from build123d import *

# Parameters (mm, degrees)
SKETCH_1_W            = 20
SKETCH_1_H            = 25
EXTRUDE_1_DEPTH       = 2
SKETCH_2_W            = 18.5
SKETCH_2_H            = 6
EXTRUDE_2_DEPTH       = 15
SKETCH_3_W            = 10
SKETCH_3_H            = 12
CUT_EXTRUDE_1_DEPTH   = 30.618406439
HOLE_WIZARD_3_0_3_1_D = 3


with BuildPart() as part:
    # 草圖1 → 填料-伸長1 (new body)
    with BuildSketch(Plane.XZ.offset(2)):
        with Locations((0, 11)):
            Rectangle(SKETCH_1_W, SKETCH_1_H)
    extrude(amount=-EXTRUDE_1_DEPTH)

    # 草圖2 → 填料-伸長2 (add)
    with BuildSketch(Plane(origin=(0, 0, 0), x_dir=(-1, 0, 0), z_dir=(0, 1, 0))):
        with Locations((0, 3)):
            Rectangle(SKETCH_2_W, SKETCH_2_H)
    extrude(amount=EXTRUDE_2_DEPTH)

    # 草圖3 → 除料-伸長1 (cut, through all)
    with BuildSketch(Plane(origin=(0, 0, 0), x_dir=(-1, 0, 0), z_dir=(0, 0, -1))):
        with Locations((0, 9)):
            Rectangle(SKETCH_3_W, SKETCH_3_H)
    extrude(amount=-CUT_EXTRUDE_1_DEPTH, mode=Mode.SUBTRACT)

    # Ø3.0 (3) 直徑孔1 (through all)
    with Locations(Plane(origin=(0, 0, 0), x_dir=(1, 0, 0), z_dir=(0, 1, 0))):
        with Locations((-7.5, -21), (7.5, -21)):
            Hole(HOLE_WIZARD_3_0_3_1_D / 2)


solid = part.part
The model under review builds one solid part; all positions refer to its coordinate system, in mm. A direction names the side the tool comes from. Give positions to 0.01 mm unless a question says otherwise; leave off trailing zeros. Write each loop counter-clockwise with the first axis right and the second up, starting at its lowest first coordinate (ties: lowest second). Pieces come first, ordered by that corner, then holes.
1. Draft analysis for pull direction Z (two halves, no side actions). For faces 1 (the flat face through (0, 0, 14)), 2 (the flat face through (0, 2, 0)), 3 (the cylindrical face through (-6.39, -1.01, 19.99)), state which applies: +Z half, -Z half, draft (parallel to the pull), parting line (faces both ways), or undercut.
2. Add section A-A, the plane x = 7.5. Write out the cut boundary in (y, z).
3. For P1, Ø2, axis at x = -4, y = 2, coming from the -Z side; P2, Ø5, axis at y = 6, z = 2, coming from the +X side; P3, Ø5, axis at y = 6, z = 4, coming from the -X side; P4, Ø6.5, axis at x = -2, z = 4, coming from the +Y side, all flat-tipped, find the tip position at first contact; note any pin that passes through.
4. Add section C-C, the plane y = 13. Write out the cut boundary in (x, z), plus the area to 3 significant figures.
5. Add section D-D, the plane z = 5. Write out the cut boundary in (x, y).
6. Tool access review of faces 4 (the flat face through (9.25, 7, 3)), 5 (the flat face through (-9.25, 7, 3)), 6 (the flat face through (5, 9, 3)), 7 (the flat face through (0, 2, 6)): name each direction out of +Z, -Z, +X, -X, +Y, -Y from which nothing blocks a thin tool from reaching the whole face with its end or side.
7. Wall thickness on L1, parallel to X at y = -1, z = 21; L2, parallel to X at y = 13.25, z = 5.5; L3, parallel to Z at x = 7.5, y = -1.1: over which ranges is each line inside the solid? List them lowest first.
8. Add section B-B, the plane z = 21. Write out the cut boundary in (x, y).
Worked answers:
1. face 1: draft
1. face 2: -Z half
1. face 3: undercut
2. outline: (-2, -1.5) - (0, -1.5) - (0, 0) - (15, 0) - (15, 6) - (0, 6) - (0, 19.5) - (-2, 19.5) - close; (-2, 22.5) - (0, 22.5) - (0, 23.5) - (-2, 23.5) - close
3. P1: stops at z = 0
3. P2: stops at x = 9.25
3. P3: stops at x = -9.25
3. P4: stops at y = 15
4. outline: (-9.25, 0) - (-5, 0) - (-5, 6) - (-9.25, 6) - close; (5, 0) - (9.25, 0) - (9.25, 6) - (5, 6) - close
4. area: 51.0 mm2
5. outline: (-10, -2) - (10, -2) - (10, 0) - (9.25, 0) - (9.25, 15) - (5, 15) - (5, 3) - (-5, 3) - (-5, 15) - (-9.25, 15) - (-9.25, 0) - (-10, 0) - close
6. face 4: +Z, -Z, +X, +Y
6. face 5: +Z, -Z, -X, +Y
6. face 6: +Z, -Z, +Y
6. face 7: +Z, +X, -X, +Y
7. L1: x = -10 to -9, -6 to 6, 9 to 10
7. L2: x = -9.25 to -5, 5 to 9.25
7. L3: z = -1.5 to 19.5, 22.5 to 23.5
8. outline: (-10, -2) - (-9, -2) - (-9, 0) - (-10, 0) - close; (-6, -2) - (6, -2) - (6, 0) - (-6, 0) - close; (9, -2) - (10, -2) - (10, 0) - (9, 0) - close
